```python
from build123d import *

# Parameters (mm, degrees)
SKETCH1_W           = 300
SKETCH1_H           = 300
SKETCH1_R           = 6
BOSS_EXTRUDE1_DEPTH = 5
SKETCH2_W           = 80
SKETCH2_H           = 100
BOSS_EXTRUDE2_DEPTH = 5
SKETCH3_R           = 6
CUT_EXTRUDE1_DEPTH  = 264


with BuildPart() as part:
    # Sketch1 → Boss-Extrude1 (new body)
    with BuildSketch(Plane.XY):
        Rectangle(SKETCH1_W, SKETCH1_H)
        with Locations((-120, 120)):
            Circle(SKETCH1_R, mode=Mode.SUBTRACT)
        with Locations((120, 120)):
            Circle(SKETCH1_R, mode=Mode.SUBTRACT)
        with Locations((-120, -120)):
            Circle(SKETCH1_R, mode=Mode.SUBTRACT)
        with Locations((120, -120)):
            Circle(SKETCH1_R, mode=Mode.SUBTRACT)
        with Locations((-91.715728753, 91.715728753)):
            Circle(SKETCH1_R, mode=Mode.SUBTRACT)
        with Locations((91.715728753, 91.715728753)):
            Circle(SKETCH1_R, mode=Mode.SUBTRACT)
        with Locations((-91.715728753, -91.715728753)):
            Circle(SKETCH1_R, mode=Mode.SUBTRACT)
        with Locations((91.715728753, -91.715728753)):
            Circle(SKETCH1_R, mode=Mode.SUBTRACT)
        with BuildLine():
            Line((-62.724350724, 120.707106781), (-34.440079476, 92.422835534))
            ThreePointArc((-34.440079476, 92.422835534), (-34.440079476, 83.937554159), (-42.925360851, 83.937554159))
            Line((-42.925360851, 83.937554159), (-71.209632098, 112.221825407))
            ThreePointArc((-71.209632098, 112.221825407), (-71.209632098, 120.707106781), (-62.724350724, 120.707106781))
        make_face(mode=Mode.SUBTRACT)
        with BuildLine():
            Line((71.209632098, 112.221825407), (42.925360851, 83.937554159))
            ThreePointArc((42.925360851, 83.937554159), (34.440079476, 83.937554159), (34.440079476, 92.422835534))
            Line((34.440079476, 92.422835534), (62.724350724, 120.707106781))
            ThreePointArc((62.724350724, 120.707106781), (71.209632098, 120.707106781), (71.209632098, 112.221825407))
        make_face(mode=Mode.SUBTRACT)
        with BuildLine():
            Line((-112.221825407, 71.209632098), (-83.937554159, 42.925360851))
            ThreePointArc((-83.937554159, 42.925360851), (-83.937554159, 34.440079476), (-92.422835534, 34.440079476))
            Line((-92.422835534, 34.440079476), (-120.707106781, 62.724350724))
            ThreePointArc((-120.707106781, 62.724350724), (-120.707106781, 71.209632098), (-112.221825407, 71.209632098))
        make_face(mode=Mode.SUBTRACT)
        with BuildLine():
            Line((120.707106781, 62.724350724), (92.422835534, 34.440079476))
            ThreePointArc((92.422835534, 34.440079476), (83.937554159, 34.440079476), (83.937554159, 42.925360851))
            Line((83.937554159, 42.925360851), (112.221825407, 71.209632098))
            ThreePointArc((112.221825407, 71.209632098), (120.707106781, 71.209632098), (120.707106781, 62.724350724))
        make_face(mode=Mode.SUBTRACT)
        with BuildLine():
            Line((112.221825407, -71.209632098), (83.937554159, -42.925360851))
            ThreePointArc((83.937554159, -42.925360851), (83.937554159, -34.440079476), (92.422835534, -34.440079476))
            Line((92.422835534, -34.440079476), (120.707106781, -62.724350724))
            ThreePointArc((120.707106781, -62.724350724), (120.707106781, -71.209632098), (112.221825407, -71.209632098))
        make_face(mode=Mode.SUBTRACT)
        with BuildLine():
            Line((62.724350724, -120.707106781), (34.440079476, -92.422835534))
            ThreePointArc((34.440079476, -92.422835534), (34.440079476, -83.937554159), (42.925360851, -83.937554159))
            Line((42.925360851, -83.937554159), (71.209632098, -112.221825407))
            ThreePointArc((71.209632098, -112.221825407), (71.209632098, -120.707106781), (62.724350724, -120.707106781))
        make_face(mode=Mode.SUBTRACT)
        with BuildLine():
            Line((-71.209632098, -112.221825407), (-42.925360851, -83.937554159))
            ThreePointArc((-42.925360851, -83.937554159), (-34.440079476, -83.937554159), (-34.440079476, -92.422835534))
            Line((-34.440079476, -92.422835534), (-62.724350724, -120.707106781))
            ThreePointArc((-62.724350724, -120.707106781), (-71.209632098, -120.707106781), (-71.209632098, -112.221825407))
        make_face(mode=Mode.SUBTRACT)
        with BuildLine():
            Line((-120.707106781, -62.724350724), (-92.422835534, -34.440079476))
            ThreePointArc((-92.422835534, -34.440079476), (-83.937554159, -34.440079476), (-83.937554159, -42.925360851))
            Line((-83.937554159, -42.925360851), (-112.221825407, -71.209632098))
            ThreePointArc((-112.221825407, -71.209632098), (-120.707106781, -71.209632098), (-120.707106781, -62.724350724))
        make_face(mode=Mode.SUBTRACT)
    extrude(amount=BOSS_EXTRUDE1_DEPTH)

    # Sketch2 → Boss-Extrude2 (add)
    with BuildSketch(Plane.XY.offset(5)):
        with Locations((-160, 0)):
            Rectangle(SKETCH2_W, SKETCH2_H)
        with Locations((160, 0)):
            Rectangle(SKETCH2_W, SKETCH2_H)
    extrude(amount=-BOSS_EXTRUDE2_DEPTH)

    # Sketch3 → Cut-Extrude1 (cut)
    with BuildSketch(Plane.XY.offset(5)):
        with Locations((-175, 32)):
            Circle(SKETCH3_R)
        with Locations((-175, -32)):
            Circle(SKETCH3_R)
        with Locations((175, 32)):
            Circle(SKETCH3_R)
        with Locations((175, -32)):
            Circle(SKETCH3_R)
    extrude(amount=-CUT_EXTRUDE1_DEPTH, mode=Mode.SUBTRACT)


solid = part.part
```
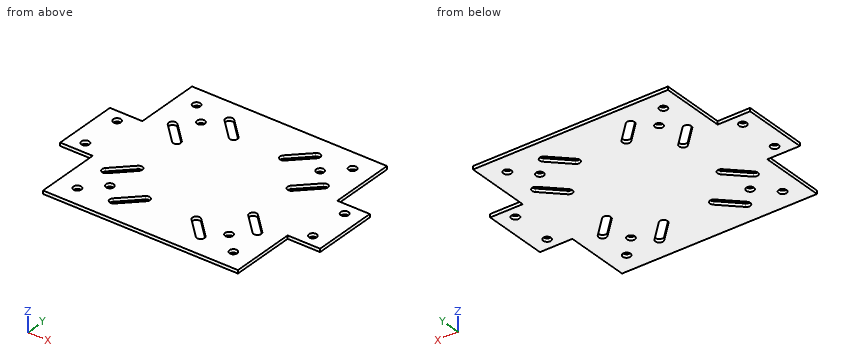
Source: CAD feature listing. Evaluate the final solid. Frame: model axes, mm. Round coordinates to 2 decimals unless told otherwise and drop trailing zeros. Loops run counter-clockwise (first coordinate to the right, second up) from the corner with the lowest first, then second, coordinate; pieces in that order, holes last. Notation, with made-up numbers: (-10.75, 50.5) - (39.25, 50.5) arc R29 cw to (39.25, 82.5) - close; hole circle Ø8 at (83.25, 60). An arc over 180 degrees is marked (long way). Use CSV: the item, a comma, the result in double quotes.
Q1. Ray query, line 1 along Y through (x, z) = (175, 1.8); line 2 along Y through (x, z) = (171, 3.45); line 3 along Y through (x, z) = (92.5, 4.25). Return the intervals inside material, ascending.
Reported:
line 1,"-50 to -38, -26 to 26, 38 to 50"
line 2,"-50 to -36.47, -27.53 to 27.53, 36.47 to 50"
line 3,"-150 to -97.66, -85.77 to -51.49, -34.52 to 34.52, 51.49 to 85.77, 97.66 to 150"
Q2. Section query C-C, the plane z = 3.4. Give the number of separate pieces and of enclosed holes in the cut face, then the cut area to 3 significant figures.
Reported:
separate pieces,"1"
enclosed holes,"20"
area,"93,900 mm^2"
Q3. Pin query (flat end, axial travel): pin 1 Ø2 at (x, y) = (13.5, 37) entering from -Z; pin 2 Ø11 at (x, y) = (-120, 120) entering from -Z; pin 3 Ø1 at (y, z) = (52, 3.5) entering from -X; pin 4 Ø1.5 at (y, z) = (-82.5, 2.5) entering from +X. Return the tip coordinate at first contact, or that it passes through.
Reported:
pin 1,"z = 0"
pin 2,"through"
pin 3,"x = -150"
pin 4,"x = 150"
Q4. Section query A-A, the plane x = 175. Output: boundary loops of the cut face in (y, z).
Reported:
outline,"(-50, 0) - (-38, 0) - (-38, 5) - (-50, 5) - close; (-26, 0) - (26, 0) - (26, 5) - (-26, 5) - close; (38, 0) - (50, 0) - (50, 5) - (38, 5) - close"
Q5. Section query B-B, the plane y = -102. Output: boundary loops of the cut face in (x, z), then the cut area to 3 significant figures.
Reported:
outline,"(-150, 0) - (-60.99, 0) - (-60.99, 5) - (-150, 5) - close; (-44.02, 0) - (44.02, 0) - (44.02, 5) - (-44.02, 5) - close; (60.99, 0) - (150, 0) - (150, 5) - (60.99, 5) - close"
area,"1,330 mm^2"
